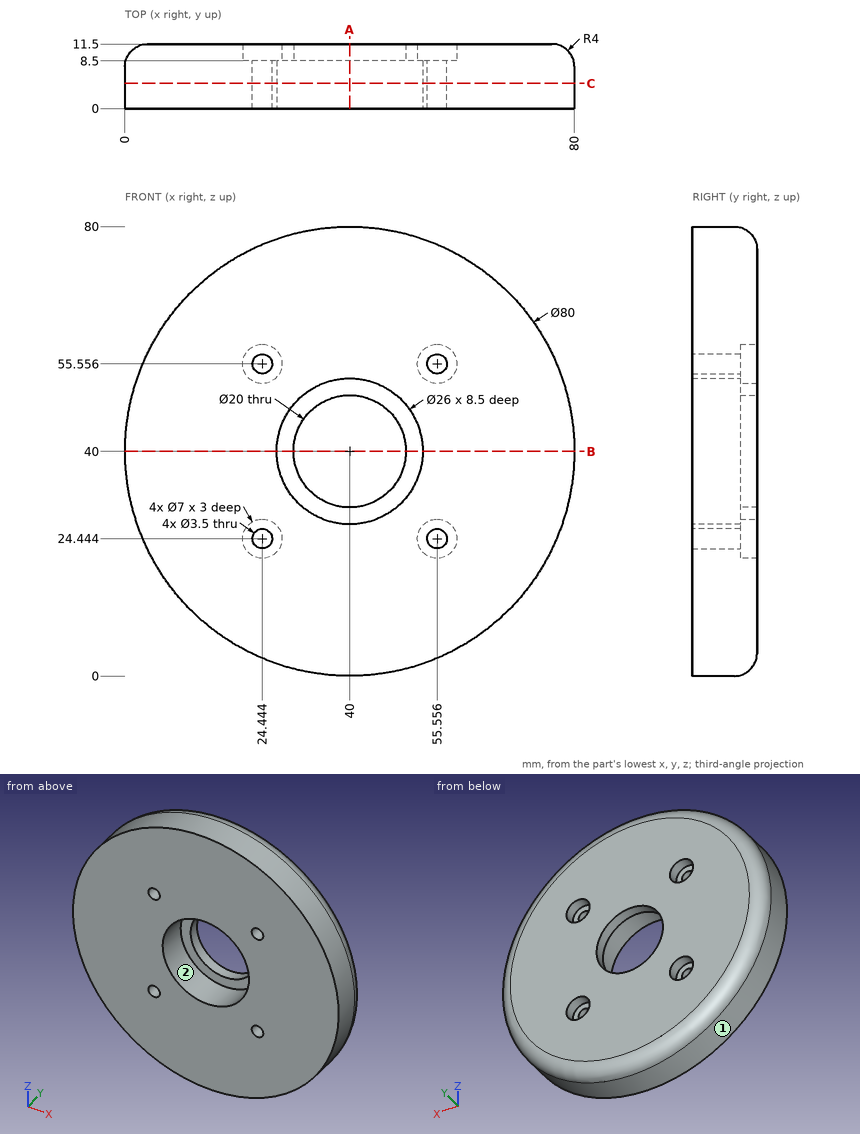
Input: dimensioned drawing with shaded views. Units: mm. Origin: part minimum x, y, z. A direction names the side the tool comes from. Give positions to 0.01 mm unless a question says otherwise; leave off trailing zeros. Loops run counter-clockwise (first coordinate to the right, second up) from the corner with the lowest first, then second, coordinate; pieces in that order, holes last. Notation, with made-up numbers: (-17, 25) - (-2, 25) arc R23 ccw to (-2, 63) - close; hole circle Ø11 at (19.25, 69). An arc over 180 degrees is marked (long way). Answer as CSV lines item,"result". Start each with the question number.
(1) Section query C-C (y = 4.5). Output: boundary loops of the cut face in (x, z).
(2) Section query A-A (x = 40). Output: boundary loops of the cut face in (y, z), and give its area (3 significant figures).
(3) Section query B-B (z = 40). Output: boundary loops of the cut face in (x, y), and give its area (3 significant figures).
(4) Reachability of the marked faces 1 and 2 from +Z, -Z, +X, -X, +Y, -Y: full face, straight path, thin tool, end or side. Return the list, or none.
(5) Ray query, line 1 along X through (y, z) = (6.25, 40); line 2 along Y through (x, z) = (35, 50.5); line 3 along X through (y, z) = (10.5, 24) (1 decimal). Return the intervals inside material, ascending. Write a range as [from, to].
(6) Pin query (flat end, axial travel): P1, Ø3, axis at x = 24.44, z = 55.56, coming from the -Y side; P2, Ø10, axis at x = 44.5, z = 46, coming from the -Y side; P3, Ø4, axis at x = 55.56, z = 24.44, coming from the +Y side; P4, Ø5, axis at x = 65, y = 7, coming from the +Z side. Return the tip coordinate at first contact, or that it passes through.
Worked answers:
1,outline,"circle Ø80 at (40, 40); hole circle Ø3.5 at (24.44, 24.44); hole circle Ø3.5 at (24.44, 55.56); hole circle Ø26 at (40, 40); hole circle Ø3.5 at (55.56, 24.44); hole circle Ø3.5 at (55.56, 55.56)"
2,outline,"(0, 0) - (7.5, 0) arc R4 ccw to (11.5, 4) - (11.5, 30) - (8.5, 30) - (8.5, 27) - (0, 27) - close; (0, 53) - (8.5, 53) - (8.5, 50) - (11.5, 50) - (11.5, 76) arc R4 ccw to (7.5, 80) - (0, 80) - close"
2,area,"632 mm^2"
3,outline,"(0, 0) - (27, 0) - (27, 8.5) - (30, 8.5) - (30, 11.5) - (4, 11.5) arc R4 ccw to (0, 7.5) - close; (50, 8.5) - (53, 8.5) - (53, 0) - (80, 0) - (80, 7.5) arc R4 ccw to (76, 11.5) - (50, 11.5) - close"
3,area,"632 mm^2"
4,face 1,"+Y, -Y"
4,face 2,"-Y"
5,line 1,"x = [0, 27], [53, 80]"
5,line 2,"y = [8.5, 11.5]"
5,line 3,"x = [4.8, 21], [27.9, 52.1], [59, 75.2]"
6,P1,"passes through"
6,P2,"stops at y = 8.5"
6,P3,"stops at y = 8.5"
6,P4,"stops at z = 73.07"
